Source: three-view drawing plus pictorial views. Frame: mm from the lowest corner of the part. Give positions to 0.01 mm unless a question says otherwise; leave off trailing zeros. Loops run counter-clockwise (first coordinate to the right, second up) from the corner with the lowest first, then second, coordinate; pieces in that order, holes last. Notation, with made-up numbers: M 57,-21.75 L 101,-21.75 A16 ccw 101,5.25 Z; hole C -19,4 d2. An arc over 180 degrees is marked long. Answer as a JSON object with one key per item and string values. Group by question number.
1) Section query C-C on z = 218.5. Return loops of the section in (x, y) (3 decimals).
2) Ray query, L1, parallel to Y at x = 18.5, z = 57.5 (3 decimals). Return the intervals inside material, ascending.
3) Section query A-A on y = 10.25. Return loops of the section in (x, z) (3 decimals), plus the area to 3 significant figures.
4) Draft query along X for the marked faces 1, 2 and 3. Return one class per face: +X half, -X half, draft (parallel to the pull), parting line (faces both ways), or undercut.
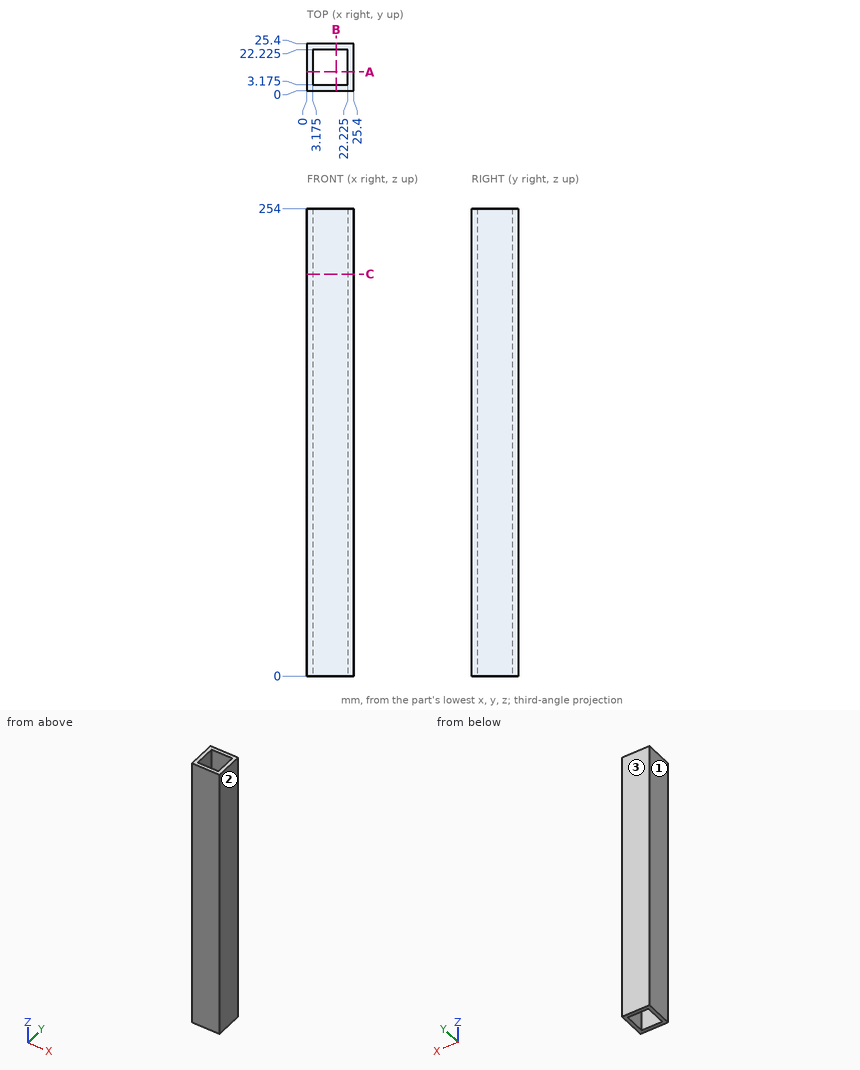
Output:
{
 "1": {"outline": "M 0,0 L 25.4,0 L 25.4,25.4 L 0,25.4 Z; hole M 3.175,3.175 L 22.225,3.175 L 22.225,22.225 L 3.175,22.225 Z"},
 "2": {"L1": "y = 0 to 3.175, 22.225 to 25.4"},
 "3": {"outline": "M 0,0 L 3.175,0 L 3.175,254 L 0,254 Z; M 22.225,0 L 25.4,0 L 25.4,254 L 22.225,254 Z", "area": "1,610 mm^2"},
 "4": {"face 1": "-X half", "face 2": "+X half", "face 3": "draft"}
}
